Source: CAD feature listing. Evaluate the final solid. Frame: model axes, mm. Face numbers are marked on the shaded views. Round coordinates to 2 decimals unless told otherwise and drop trailing zeros. Write each loop counter-clockwise with the first axis right and the second up, starting at its lowest first coordinate (ties: lowest second). Pieces come first, ordered by that corner, then holes. Notation, with made-up numbers: M 65.5,54 L 91.5,54 A23 cw 91.5,88 Z; hole C 33,54.5 d3. An arc over 180 degrees is marked long. Use a Markdown table: item, result.
```python
from build123d import *

# Parameters (mm, degrees)
SKETCH2_R           = 1.6
BOSS_EXTRUDE1_DEPTH = 3
SKETCH3_R           = 3.5
SKETCH3_R_2         = 2.75
BOSS_EXTRUDE2_DEPTH = 2


with BuildPart() as part:
    # Sketch2 → Boss-Extrude1 (new body)
    with BuildSketch(Plane.XY):
        with BuildLine():
            ThreePointArc((-15.83772234, 1.5), (-22.5, 0), (-15.83772234, -1.5))
            ThreePointArc((-15.83772234, -1.5), (0, -4.768997412), (15.83772234, -1.5))
            ThreePointArc((15.83772234, -1.5), (22.5, 0), (15.83772234, 1.5))
            ThreePointArc((15.83772234, 1.5), (0, -1.768997412), (-15.83772234, 1.5))
        make_face()
        with Locations((-19, 0)):
            Circle(SKETCH2_R, mode=Mode.SUBTRACT)
        with Locations((19, 0)):
            Circle(SKETCH2_R, mode=Mode.SUBTRACT)
    extrude(amount=BOSS_EXTRUDE1_DEPTH)

    # Sketch3 → Boss-Extrude2 (add)
    with BuildSketch(Plane.XY.offset(3)):
        with Locations(Location((19, 0, 0), (0, 0, 154.623066475))):
            Circle(SKETCH3_R)
        with Locations((19, 0)):
            Circle(SKETCH3_R_2, mode=Mode.SUBTRACT)
    extrude(amount=BOSS_EXTRUDE2_DEPTH)


solid = part.part
```
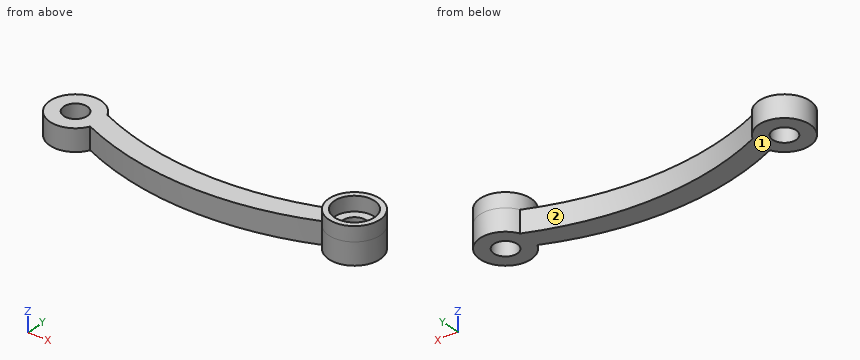
Q1. Section D-D on z = 0.45. Return loops of the section in (x, y).
Results are:
| item | result |
|---|---|
| outline | M -15.84,-1.5 A40 ccw 15.84,-1.5 A3.5 ccw long 15.84,1.5 A40 cw -15.84,1.5 A3.5 ccw long Z; hole C -19,0 d3.2; hole C 19,0 d3.2 |
Q2. First-contact query: pin 1 Ø2 at (x, y) = (-9, 0) entering from +Z; pin 2 Ø1 at (y, z) = (2.5, 1) entering from +X; pin 3 Ø1.5 at (x, z) = (11.5, 2.5) entering from -Y. Flat tips, straight axial feed; report the tip coordinate or a pass-through.
Results are:
| item | result |
|---|---|
| pin 1 | z = 3 |
| pin 2 | x = 21.87 |
| pin 3 | y = -3.3 |
Q3. Section C-C on z = 3.4. Return loops of the section in (x, y).
Results are:
| item | result |
|---|---|
| outline | C 19,0 d7; hole C 19,0 d5.5 |
Q4. Section A-A on x = -19. Return loops of the section in (y, z).
Results are:
| item | result |
|---|---|
| outline | M -3.5,0 L -1.6,0 L -1.6,3 L -3.5,3 Z; M 1.6,0 L 3.5,0 L 3.5,3 L 1.6,3 Z |
Q5. Mould query, pull axis X, two halves, no side actions, for the marked faces 1 and 2. Classes: +X half, -X half, draft (parallel to the pull), parting line (faces both ways), or undercut.
Results are:
| item | result |
|---|---|
| face 1 | draft |
| face 2 | undercut |
Q6. Section B-B on y = 2. Return loops of the section in (x, z).
Results are:
| item | result |
|---|---|
| outline | M -21.87,0 L -16.13,0 L -16.13,3 L -21.87,3 Z; M 16.13,0 L 21.87,0 L 21.87,5 L 20.89,5 L 20.89,3 L 17.11,3 L 17.11,5 L 16.13,5 Z |
Q7. Line query: L1, parallel to Y at x = 19, z = 3.75; L2, parallel to Y at x = 19, z = 1.2; L3, parallel to Z at x = -1, y = -2.25. Output: solid intervals per line, ascending.
Results are:
| item | result |
|---|---|
| L1 | -3.5 to -2.75, 2.75 to 3.5 |
| L2 | -3.5 to -1.6, 1.6 to 3.5 |
| L3 | 0 to 3 |
